Autodesk Inventor part; units mm, degrees
ref_plane "Work Plane1" through (0, 0, 58.5) normal (0, 0, 1) x (1, 0, 0)
ref_plane "YZ Plane" through (0, 0, 0) normal (1, 0, 0) x (0, 1, 0)
ref_plane "XZ Plane" through (0, 0, 0) normal (0, 1, 0) x (-1, 0, 0)
sketch "Sketch1" plane through (0, 0, 0) normal (0, 0, 1) x (1, 0, 0)
  line L0 (-100, 57.735) -> (0, 115.4701)
  line L1 (0, 115.4701) -> (100, 57.735)
  line L2 (100, 57.735) -> (100, -57.735)
  line L3 (100, -57.735) -> (0, -115.4701)
  line L4 (0, -115.4701) -> (-100, -57.735)
  line L5 (-100, -57.735) -> (-100, 57.735)
  line L6 (-95, 54.8483) -> (0, 109.6966)
  line L7 (0, 109.6966) -> (95, 54.8483)
  line L8 (95, 54.8483) -> (95, -54.8483)
  line L9 (95, -54.8483) -> (0, -109.6966)
  line L10 (0, -109.6966) -> (-95, -54.8483)
  line L11 (-95, -54.8483) -> (-95, 54.8483)
  line L12 (-100, -57.735) -> (0, 0)
  line L13 (0, 0) -> (0, -115.4701)
  line L14 (100, -57.735) -> (0, 0)
  line L15 (100, 57.735) -> (0, 0)
  line L16 (0, 115.4701) -> (0, 0)
  line L17 (-100, 57.735) -> (0, 0)
  line L18 (0, -109.6966) -> (0, 0)
  line L19 (95, -54.8483) -> (0, 0)
  line L20 (95, 54.8483) -> (0, 0)
  line L21 (0, 109.6966) -> (0, 0)
  line L22 (-95, 54.8483) -> (0, 0)
  line L23 (-95, -54.8483) -> (0, 0)
  dimension "d0" = 200
  dimension "d1" = 190
ref_plane "Work Plane1" through (0, 0, 58.5) normal (0, 0, 1) x (1, 0, 0)
sketch "Sketch2" plane through (0, 0, 58.5) normal (0, 0, 1) x (1, 0, 0)
  point P0 (0, 0)
  point P1 (0, 0)
extrude "Extrusion1" add sketch "Sketch1" along normal up to surface (58.5 mm away)
loft "Loft1" cut keep common part section 1 edges at (-50, -86.6025, 0) (-100, 0, 0) (-50, 86.6025, 0) (50, 86.6025, 0) (100, 0, 0) (50, -86.6025, 0) section 2 point at (0, 0, 58.5)
shell "Shell1" thickness 10 removed faces 1 at (0, 0, 0)
sketch "Sketch4" plane through (0, 0, 0) normal (0, 0, -1) x (-1, 0, 0)
  line L0 (0, -92.6022) -> (-80.1958, -46.3011)
  line L1 (0, -92.6022) -> (-80.1958, -46.3011)
  line L2 (-80.1958, -46.3011) -> (-80.1958, 46.3011)
  line L3 (-80.1958, 46.3011) -> (0, 92.6022)
  line L4 (0, 92.6022) -> (80.1958, 46.3011)
  line L5 (80.1958, 46.3011) -> (80.1958, -46.3011)
  line L6 (80.1958, -46.3011) -> (0, -92.6022)
  line L7 (0, -95.8401) -> (-83, -47.9201)
  line L8 (-83, -47.9201) -> (-83, 47.9201)
  line L9 (-83, 47.9201) -> (0, 95.8401)
  line L10 (0, 95.8401) -> (83, 47.9201)
  line L11 (83, 47.9201) -> (83, -47.9201)
  line L12 (83, -47.9201) -> (0, -95.8401)
  line L13 (83, -47.9201) -> (80.1958, -46.3011)
  line L14 (0, -95.8401) -> (0, -92.6022)
  line L15 (-83, -47.9201) -> (-80.1958, -46.3011)
  line L16 (-83, 47.9201) -> (-80.1958, 46.3011)
  line L17 (0, 95.8401) -> (0, 92.6022)
  line L18 (80.1958, 46.3011) -> (83, 47.9201)
  point P0 (0, 0)
  point P1 (0, 0)
  point P2 (0, 0)
  dimension "d18" = 166
extrude "Extrusion3" add sketch "Sketch4" along normal blind 20 contours L14 L7 L15 L0 | L6 L13 L12 L14 | L15 L8 L16 L2 | L5 L18 L11 L13 | L16 L9 L17 L3 | L4 L17 L10 L18
properties part number "Phage_Hat"
The model under review builds one solid part; all positions refer to its coordinate system, in mm. A direction names the side the tool comes from. Coordinates: 2 decimals unless noted, no trailing zeros. Write each loop counter-clockwise with the first axis right and the second up, starting at its lowest first coordinate (ties: lowest second). Pieces come first, ordered by that corner, then holes.
1) To check wall thickness, follow probe 1 along X at (y, z) = (78, -16.5); probe 2 along Y at (x, z) = (-17.5, 27); probe 3 along X at (y, z) = (-85, -5). State the ranges of each line that lie inside material, in increasing order.
2) The part is to be moulded in two halves that separate along Y. For faces 1 (the face through (48.4, -0.6, 18.6)), 2 (the face through (30.91, 51.91, 23.16)), 3 (the face through (-83, 1, -10)), say which applies: pulls with the +Y half, pulls with the -Y half, needs draft (parallel to the pull), parting line crosses it, or undercut.
3) We need section C-C on y = -79.5. State the section outline as (x, z) points.
4) Machinability: for faces 4 (the face through (40.919, -72.216, -9.86)), 5 (the face through (60.41, -0.81, 23.16)), 6 (the face through (-40.919, 72.216, -9.86)), 7 (the face through (-40.659, -69.128, -9.86)), which of the approach directions +Z, -Z, +X, -X, +Y, -Y give a long, thin tool a straight path to every point of the face, cutting with its end or side? Answer none if there is none.
5) We need section B-B on x = -44. State the section outline as (y, z) points.
6) We need section A-A on z = -3. State the section outline as (x, y) points, then the cut area to 3 significant figures.
7) Clearance check with flat-ended pins moving along their axes: pin 1 Ø4 at (y, z) = (25, 29.5) entering from +X; pin 2 Ø6 at (y, z) = (16, -12.5) entering from +X; pin 3 Ø5 at (x, y) = (-5, -23.5) entering from +Z. State where each tip first meets the part, or that it passes through.
8) We need section D-D on z = 31. State the section outline as (x, y) points.
Answer list:
1. probe 1: x = -30.9 to -25.29, 25.29 to 30.9
1. probe 2: y = -52.07 to -29.2, 29.2 to 52.07
1. probe 3: x = -18.78 to -13.17, 13.17 to 18.78
2. face 1: undercut
2. face 2: pulls with the +Y half
2. face 3: needs draft
3. outline: (-62.3, 0) - (-28.3, 0) - (-28.3, -20) - (-22.69, -20) - (-22.69, 0) - (0, 6.64) - (22.69, 0) - (22.69, -20) - (28.3, -20) - (28.3, 0) - (62.3, 0) - (0, 18.22) - close
4. face 4: -Z, +X, -Y
4. face 5: +Z, +X, +Y, -Y
4. face 6: -Z, -X, +Y
4. face 7: -Z
5. outline: (-90.07, 0) - (-70.44, 0) - (-70.44, -20) - (-67.2, -20) - (-67.2, 0) - (-25.4, 21.17) - (25.4, 21.17) - (67.2, 0) - (67.2, -20) - (70.44, -20) - (70.44, 0) - (90.07, 0) - (25.4, 32.76) - (-25.4, 32.76) - close
6. outline: (-83, -47.92) - (0, -95.84) - (83, -47.92) - (83, 47.92) - (0, 95.84) - (-83, 47.92) - close; hole (-80.2, -46.3) - (0, -92.6) - (80.2, -46.3) - (80.2, 46.3) - (0, 92.6) - (-80.2, 46.3) - close
6. area: 1,590 mm2
7. pin 1: stops at x = 52.99
7. pin 2: stops at x = 83
7. pin 3: stops at z = 46.59
8. outline: (-47.01, -27.14) - (0, -54.28) - (47.01, -27.14) - (47.01, 27.14) - (0, 54.28) - (-47.01, 27.14) - close; hole (-27.2, -15.71) - (0, -31.41) - (27.2, -15.71) - (27.2, 15.71) - (0, 31.41) - (-27.2, 15.71) - close
